The listing builds one solid part. Answer for the finished solid, in the listing's coordinates (mm). Coordinates: 2 decimals unless noted, no trailing zeros. Order: outer loops, then holes, each group sorted by start corner. A loop starts at its lowest first (then second) coordinate and runs counter-clockwise, first axis right, second up. Notation, with made-up numbers: (-17, 9) -> (9, 9) arc R29 cw to (9, 47) -> close; hole circle Ø6 at (30.5, -22.5). An arc over 180 degrees is marked (long way). Return JSON: item names as keys, results as strings.
from build123d import *

# Parameters (mm, degrees)
SKETCH1_R           = 60
BOSS_EXTRUDE1_DEPTH = 5
SKETCH2_R           = 1.5
CUT_EXTRUDE1_DEPTH  = 5
CUT_EXTRUDE2_REACH  = 87
SKETCH3_R           = 1.5


with BuildPart() as part:
    # Sketch1 → Boss-Extrude1 (new body)
    with BuildSketch(Plane(origin=(0, 0, 0), x_dir=(1, 0, 0), z_dir=(0, 1, 0))):
        with Locations(Location((0, 0, 0), (0, 0, 270))):
            Circle(SKETCH1_R)
    extrude(amount=BOSS_EXTRUDE1_DEPTH)

    # Sketch2 → Cut-Extrude1 (cut)
    with BuildSketch(Plane(origin=(0, 5, 0), x_dir=(1, 0, 0), z_dir=(0, 1, 0))):
        with Locations(Location((45, 0, 0), (0, 0, 270))):
            Circle(SKETCH2_R)
        with Locations(Location((0, -45, 0), (0, 0, 270))):
            Circle(SKETCH2_R)
        with Locations(Location((-45, 0, 0), (0, 0, 270))):
            Circle(SKETCH2_R)
        with Locations(Location((0, 45, 0), (0, 0, 270))):
            Circle(SKETCH2_R)
    extrude(amount=-CUT_EXTRUDE1_DEPTH, mode=Mode.SUBTRACT)

    # Sketch3 → Cut-Extrude2 (cut, up to next)
    with BuildSketch(Plane(origin=(0, 5, 0), x_dir=(1, 0, 0), z_dir=(0, 1, 0)), mode=Mode.PRIVATE) as cut_extrude2_sk1:
        with Locations(Location((0, -8, 0), (0, 0, 270))):
            Circle(SKETCH3_R)
    cut_extrude2_tool1 = extrude(cut_extrude2_sk1.sketch, amount=-CUT_EXTRUDE2_REACH, mode=Mode.PRIVATE) & part.part
    # Sketch3 → Cut-Extrude2 (cut, up to next)
    with BuildSketch(Plane(origin=(0, 5, 0), x_dir=(1, 0, 0), z_dir=(0, 1, 0)), mode=Mode.PRIVATE) as cut_extrude2_sk2:
        with Locations(Location((0, 8, 0), (0, 0, 270))):
            Circle(SKETCH3_R)
    cut_extrude2_tool2 = extrude(cut_extrude2_sk2.sketch, amount=-CUT_EXTRUDE2_REACH, mode=Mode.PRIVATE) & part.part
    add(cut_extrude2_tool1.solids().sort_by_distance((0, 5, 8))[0], mode=Mode.SUBTRACT)
    add(cut_extrude2_tool2.solids().sort_by_distance((0, 5, -8))[0], mode=Mode.SUBTRACT)


solid = part.part
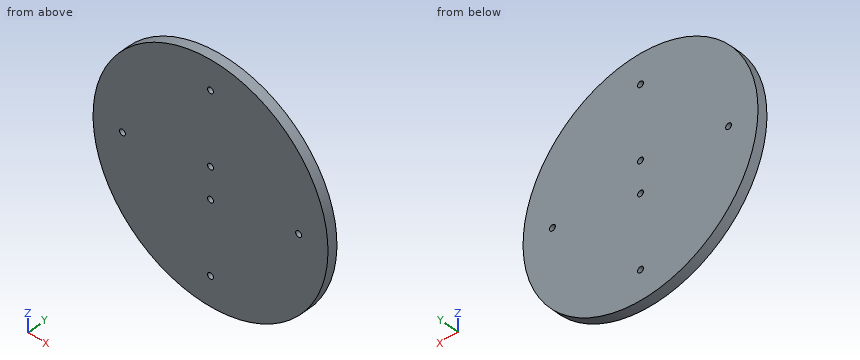
1. The part is cut by section B-B on y = 2.2. Give the vertices of the cut face in (x, z), and give its area (3 significant figures).
Answer block:
{"outline": "circle Ø120 at (0, 0); hole circle Ø3 at (-45, 0); hole circle Ø3 at (0, -45); hole circle Ø3 at (0, -8); hole circle Ø3 at (0, 8); hole circle Ø3 at (0, 45); hole circle Ø3 at (45, 0)", "area": "11,300 mm2"}
2. The part is cut by section D-D on x = -11. Give the vertices of the cut face in (y, z), and give its area (3 significant figures).
Answer block:
{"outline": "(0, -58.98) -> (5, -58.98) -> (5, 58.98) -> (0, 58.98) -> close", "area": "590 mm2"}
3. Each of these flat-tipped pins is pushed along its axis until it touches: pin 1 Ø2 at (x, y) = (-15, 1) entering from -Z; pin 2 Ø2 at (x, y) = (-10, 3) entering from +Z; pin 3 Ø2 at (y, z) = (2, -6) entering from +X. Where does it stop, or does it pass through?
Answer block:
{"pin 1": "stops at z = -58.34", "pin 2": "stops at z = 59.32", "pin 3": "stops at x = 59.79"}
4. The part is cut by section A-A on z = 0. Give the vertices of the cut face in (x, y).
Answer block:
{"outline": "(-60, 0) -> (-46.5, 0) -> (-46.5, 5) -> (-60, 5) -> close; (-43.5, 0) -> (43.5, 0) -> (43.5, 5) -> (-43.5, 5) -> close; (46.5, 0) -> (60, 0) -> (60, 5) -> (46.5, 5) -> close"}
5. The part is cut by section C-C on x = -45. Give the vertices of the cut face in (y, z).
Answer block:
{"outline": "(0, -39.69) -> (5, -39.69) -> (5, -1.5) -> (0, -1.5) -> close; (0, 1.5) -> (5, 1.5) -> (5, 39.69) -> (0, 39.69) -> close"}
6. Consider line 1 (X direction, y = 3.3, z = 0); line 2 (X direction, y = 3.7, z = -1); line 3 (X direction, y = 3.9, z = 8). Determine where each line is inside the solid, lowest interval first. Write a range as from..to.
Answer block:
{"line 1": "x = -60..-46.5, -43.5..43.5, 46.5..60", "line 2": "x = -59.99..-46.12, -43.88..43.88, 46.12..59.99", "line 3": "x = -59.46..-1.5, 1.5..59.46"}
